Input: part model. Units: mm. Frame: model coordinates. Face numbers are marked on the shaded views. A direction names the side the tool comes from. Coordinates: 2 decimals unless noted, no trailing zeros. Loops run counter-clockwise (first coordinate to the right, second up) from the corner with the lowest first, then second, coordinate; pieces in that order, holes last.
(1) Line query: L1, parallel to X at y = 140, z = -1245; L2, parallel to Y at x = -100, z = -1242; L3, parallel to Z at x = -1586, y = 467. Output: solid intervals per line, ascending.
(2) Section B-B, the plane y = 411.5. Return loops of the section in (x, z), then the cut area to 3 significant figures.
(3) Set-up query: the marked faces 4 and 5. Return all of +Z, -Z, +X, -X, +Y, -Y with unobstructed straight access to the full face (end or side cutting, diameter ignored); none if empty.
(4) Section C-C, the plane z = -787.5. Return loops of the section in (x, y).
(5) Mould query, pull axis X, two halves, no side actions, for the marked faces 1, 2 and 3. Classes: released by +X, released by -X, zero draft, split by the parting line, or undercut.
(6) Section A-A, the plane x = -1414.5. Return loops of the section in (y, z).
(7) Contact query for flat-ended pins moving along their axis: P1, Ø7, axis at x = -2400, y = 100, coming from the -Z side; P2, Ø3, axis at x = -2440, y = 17.5, coming from the +Z side; P3, Ø15, axis at x = -14, z = -137.5, coming from the -Y side. Output: stop coordinate, or through.
Autodesk Inventor part; units mm, degrees
ref_plane "Work Plane1" through (-2500, 0, -625) normal (0, 0, 1) x (1, 0, 0)
ref_plane "Work Plane2" through (-1250, 0, -1250) normal (-1, 0, 0) x (0, 0, 1)
ref_plane "YZ Plane" through (0, 0, 0) normal (1, 0, 0) x (0, 1, 0)
sketch "Sketch1" plane through (0, 0, 0) normal (0, 1, 0) x (-1, 0, 0)
  line L0 (0, 0) -> (2500, 0)
  line L1 (2500, 0) -> (2500, -1250)
  line L2 (2500, -1250) -> (0, -1250)
  line L3 (0, -1250) -> (0, 0)
  dimension "d0" = 2500
  dimension "d1" = 1250
extrude "Extrusion1" add sketch "Sketch1" along normal blind 600
sketch "Sketch2" plane through (0, 0, 0) normal (0, -1, 0) x (1, 0, 0)
  line L0 (-50, -50) -> (-2450, -50)
  line L1 (-2450, -50) -> (-2450, -1200)
  line L2 (-2450, -1200) -> (-50, -1200)
  line L3 (-50, -1200) -> (-50, -50)
  line L4 (0, 0) -> (-2500, 0)
  line L5 (0, -1250) -> (0, 0)
  dimension "d4" = 2400
  dimension "d5" = 1150
  dimension "d8" = 50
  dimension "d9" = 50
  dimension "d10" = 2500
  dimension "d11" = 1250
extrude "Extrusion2" cut sketch "Sketch2" against normal blind 500
sketch "Sketch3" plane through (-2500, 0, 0) normal (0, 0, 1) x (1, 0, 0)
  line L0 (2500, 0) -> (0, 0)
  line L1 (2500, 0) -> (2500, 600)
  line L2 (0, 0) -> (0, 600)
  circle A0 centre (2440, 18) radius 3
  circle A1 centre (2420, 18) radius 3
  circle A2 centre (2400, 100) radius 4.25
  circle A3 centre (2400, 140.5) radius 4.25
  dimension "d12" = 6
  dimension "d13" = 18
  dimension "d14" = 60
  dimension "d20" = 6
  dimension "d21" = 18
  dimension "d23" = 20
  dimension "d24" = 8.5
  dimension "d25" = 8.5
  dimension "d26" = 100
  dimension "d27" = 40.5
  dimension "d28" = 100
  dimension "d29" = 100
extrude "Extrusion3" cut sketch "Sketch3" against normal blind 10
ref_plane "Work Plane1" through (-2500, 0, -625) normal (0, 0, 1) x (1, 0, 0)
mirror "Mirror1" about plane through (-2500, 0, -625) normal (0, 0, 1) of "Extrusion3"
ref_plane "Work Plane2" through (-1250, 0, -1250) normal (-1, 0, 0) x (0, 0, 1)
mirror "Mirror2" about plane through (-1250, 0, -1250) normal (-1, 0, 0) of "Extrusion3"
mirror "Mirror3" about plane through (-2500, 0, -625) normal (0, 0, 1) of "Mirror2", "Extrusion3"
sketch "Sketch4" plane through (0, 0, 0) normal (0, -1, 0) x (1, 0, 0)
  circle A0 centre (-25, -150) radius 25
  line L0 (0, 0) -> (-2500, 0)
  line L1 (0, -1250) -> (0, 0)
  circle A1 centre (-2475, -150) radius 25
  circle A2 centre (-25, -1100) radius 25
  circle A3 centre (-2475, -1100) radius 25
  dimension "d30" = 50
  dimension "d31" = 25
  dimension "d32" = 150
  dimension "d33" = 2500
  dimension "d34" = 1250
  dimension "d37" = 2450
  dimension "d40" = 950
extrude "Extrusion4" cut sketch "Sketch4" against normal blind 10
equation "\"d4\" = d10 - 2 * d9"
equation "\"d5\" = d11 - 2 * d8"
equation "\"d9\" = d8"
equation "\"d13\" = 3 * d12"
equation "\"d21\" = d13"
equation "\"d29\" = d28"
equation "\"d37\" = d33 - 2 * d31"
equation "\"d40\" = d34 - 2 * d32"
properties part number "Base" material "Wood (Birch)"
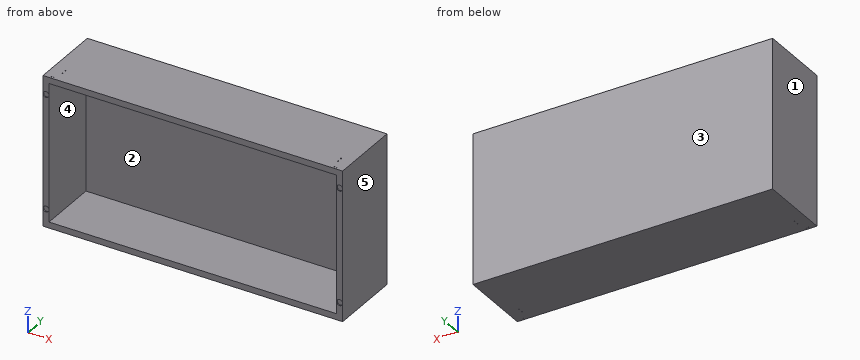
Report:
1. L1: x = -2500 to -2404.22, -2395.78 to -104.22, -95.78 to 0
1. L2: y = 0 to 95.75, 104.25 to 136.25, 144.75 to 600
1. L3: z = -1250 to -1200, -50 to 0
2. outline: (-2500, -1250) - (0, -1250) - (0, 0) - (-2500, 0) - close; hole (-2450, -1200) - (-50, -1200) - (-50, -50) - (-2450, -50) - close
2. area: 365,000 mm2
3. face 4: -Y
3. face 5: +Z, -Z, +X, +Y, -Y
4. outline: (-2500, 0) - (-2450, 0) - (-2450, 500) - (-50, 500) - (-50, 0) - (0, 0) - (0, 600) - (-2500, 600) - close
5. face 1: released by -X
5. face 2: undercut
5. face 3: zero draft
6. outline: (0, -1250) - (600, -1250) - (600, 0) - (0, 0) - (0, -50) - (500, -50) - (500, -1200) - (0, -1200) - close
7. P1: stops at z = -1240
7. P2: stops at z = -10
7. P3: stops at y = 10
